Geometry: final body of the model. Coordinates: model frame, mm. A direction names the side the tool comes from. Give positions to 0.01 mm unless a question says otherwise; leave off trailing zeros. Order: outer loops, then holes, each group sorted by start corner. A loop starts at its lowest first (then second) coordinate and runs counter-clockwise, first axis right, second up. Notation, with made-up numbers: M 6.25,57 L 39.25,57 A12 cw 39.25,71 Z; hole C 42,88 d9. An arc over 180 degrees is marked long. Write item = value, one per line. Start each with the question number.
from build123d import *

# Parameters (mm, degrees)
SKETCH_1_W                         = 182.5
SKETCH_1_H                         = 55
SM_BASE_FLANGE_1_DEPTH             = 2
SM_EDGE_FLANGE_1_STRIP_W           = 9.4732
SM_EDGE_FLANGE_1_STRIP_H           = 2
SM_EDGE_FLANGE_1_STRIP_CUT_DEPTH   = 55
SM_EDGE_FLANGE_1_STRIP_2_W         = 9.4732
SM_EDGE_FLANGE_1_STRIP_2_H         = 2
SM_EDGE_FLANGE_1_STRIP_CUT_2_DEPTH = 55
SM_EDGE_FLANGE_1_DEPTH             = 55
SM_EDGE_FLANGE_1_BEND_DEPTH        = 55
SKETCH_12_W                        = 8
SKETCH_12_H                        = 7.5
CUT_EXTRUDE_1_DEPTH                = 10
FILLET_1_R                         = 2
SKETCH_13_R                        = 1.6
CUT_EXTRUDE_2_DEPTH                = 197
SKETCH_14_R                        = 1.6
CUT_EXTRUDE_3_DEPTH                = 10


# Sheet-metal steps are written as plain solids
with BuildPart() as part:
    # Sketch 1 → Базовая кромка1 (new body)
    with BuildSketch(Plane.XY):
        Rectangle(SKETCH_1_W, SKETCH_1_H)
    extrude(amount=-SM_BASE_FLANGE_1_DEPTH)

    # Ребро-кромка1 strip (across the edge) → Ребро-кромка1 strip cut (cut)
    with BuildSketch(Plane(origin=(-91.25, 27.5, 0), x_dir=(1, 0, 0), z_dir=(0, -1, 0))):
        with Locations((-2, -1)):
            Rectangle(SM_EDGE_FLANGE_1_STRIP_W, SM_EDGE_FLANGE_1_STRIP_H)
    extrude(amount=SM_EDGE_FLANGE_1_STRIP_CUT_DEPTH, mode=Mode.SUBTRACT)

    # Ребро-кромка1 strip 2 (across the edge) → Ребро-кромка1 strip cut 2 (cut)
    with BuildSketch(Plane(origin=(91.25, -27.5, 0), x_dir=(-1, 0, 0), z_dir=(0, 1, 0))):
        with Locations((-2, -1)):
            Rectangle(SM_EDGE_FLANGE_1_STRIP_2_W, SM_EDGE_FLANGE_1_STRIP_2_H)
    extrude(amount=SM_EDGE_FLANGE_1_STRIP_CUT_2_DEPTH, mode=Mode.SUBTRACT)

    # Ребро-кромка1 section (across the edge) → Ребро-кромка1 (add)
    with BuildSketch(Plane(origin=(-91.25, 27.5, 0), x_dir=(1, 0, 0), z_dir=(0, -1, 0))):
        with BuildLine():
            Line((0, 0.7366), (0, 28))
            Line((0, 28), (2, 28))
            Line((2, 28), (2, 0.7366))
            ThreePointArc((2, 0.7366), (2.215745145, 0.215745145), (2.7366, 0))
            Line((2.7366, 0), (2.7366, -2))
            ThreePointArc((2.7366, -2), (0.801531583, -1.198468417), (0, 0.7366))
        make_face()
    extrude(amount=SM_EDGE_FLANGE_1_DEPTH)

    # Ребро-кромка1 section 2 (across the edge) → Ребро-кромка1 bend (add)
    with BuildSketch(Plane(origin=(91.25, -27.5, 0), x_dir=(-1, 0, 0), z_dir=(0, 1, 0))):
        with BuildLine():
            Line((0, 0.7366), (0, 28))
            Line((0, 28), (2, 28))
            Line((2, 28), (2, 0.7366))
            ThreePointArc((2, 0.7366), (2.215745145, 0.215745145), (2.7366, 0))
            Line((2.7366, 0), (2.7366, -2))
            ThreePointArc((2.7366, -2), (0.801531583, -1.198468417), (0, 0.7366))
        make_face()
    extrude(amount=SM_EDGE_FLANGE_1_BEND_DEPTH)

    # Эскиз12 → Вырез-Вытянуть1 (cut)
    with BuildSketch(Plane.XY):
        with Locations((0, 23.75)):
            Rectangle(SKETCH_12_W, SKETCH_12_H)
        with Locations((30, 23.75)):
            Rectangle(SKETCH_12_W, SKETCH_12_H)
        with Locations((-30, 23.75)):
            Rectangle(SKETCH_12_W, SKETCH_12_H)
        with Locations((-60, 23.75)):
            Rectangle(SKETCH_12_W, SKETCH_12_H)
    extrude(amount=-CUT_EXTRUDE_1_DEPTH, mode=Mode.SUBTRACT)

    # Скругление1
    fillet_1_edges = [part.edges().sort_by_distance(p)[0] for p in [
        (-56, 20, -1),
        (-64, 20, -1),
        (-26, 20, -1),
        (-34, 20, -1),
        (34, 20, -1),
        (26, 20, -1),
        (4, 20, -1),
        (-4, 20, -1),
    ]]
    fillet(fillet_1_edges, radius=FILLET_1_R)

    # Эскиз13 → Вырез-Вытянуть2 (cut)
    with BuildSketch(Plane(origin=(91.25, 0, 0), x_dir=(0, 0, -1), z_dir=(1, 0, 0))):
        with Locations((-20.5, -20)):
            Circle(SKETCH_13_R)
        with Locations((-20.5, 22)):
            Circle(SKETCH_13_R)
    extrude(amount=-CUT_EXTRUDE_2_DEPTH, mode=Mode.SUBTRACT)

    # Эскиз14 → Вырез-Вытянуть3 (cut)
    with BuildSketch(Plane(origin=(0, 0, -2), x_dir=(-1, 0, 0), z_dir=(0, 0, -1))):
        with Locations((-63.25, 15.5)):
            Circle(SKETCH_14_R)
        with Locations((-63.25, -9.5)):
            Circle(SKETCH_14_R)
    extrude(amount=-CUT_EXTRUDE_3_DEPTH, mode=Mode.SUBTRACT)


solid = part.part
1) Cut plane C-C (y = -9.5). Return loops of the section in (x, z).
2) Ray query, L1, parallel to Y at x = -90.75, z = 20.5; L2, parallel to X at y = 7.5, z = 23.25; L3, parallel to Z at x = -8, y = 8. Return the intervals inside material, ascending.
3) Cut plane B-B (y = -20). Return loops of the section in (x, z).
4) Draft query along X for faces 3 (the flat face through (-91.25, 0, 14)), 4 (the cylindrical face through (90.264, -18.414, 20.708)), 5 (the flat face through (-1, 0, 0)). Return one class per face: pulls with the +X half, pulls with the -X half, needs draft (parallel to the pull), parting line crosses it, or undercut.
5) Pin query (flat end, axial travel): pin 1 Ø1.9 at (x, y) = (63.25, -9.5) entering from -Z; pin 2 Ø1 at (y, z) = (24, -1.5) entering from -X; pin 3 Ø2 at (y, z) = (23.5, -1) entering from +X; pin 4 Ø1.6 at (x, z) = (-61, -1) entering from +Y. Return the tip coordinate at first contact, or that it passes through.
6) Access query for faces 1 (the cylindrical face through (90.264, 23.586, 20.708)), 2 (the flat face through (-89.25, 0, 15)). Directions: +Z, -Z, +X, -X, +Y, -Y. A direction counts if a zero-diameter tool reaches every point of the face in a straight line with its end or side. Return the directions, or none.
7) Cut plane D-D (x = 63.25). Return loops of the section in (y, z).
8) Cut plane A-A (z = 15.25). Return loops of the section in (x, y).
Reply:
q1.outline = M -91.25,0.74 A2.74 ccw -88.51,-2 L 61.65,-2 L 61.65,0 L -88.51,0 A0.74 cw -89.25,0.74 L -89.25,28 L -91.25,28 Z; M 64.85,-2 L 88.51,-2 A2.74 ccw 91.25,0.74 L 91.25,28 L 89.25,28 L 89.25,0.74 A0.74 cw 88.51,0 L 64.85,0 Z
q2.L1 = -27.5 to -21.6, -18.4 to 20.4, 23.6 to 27.5
q2.L2 = -91.25 to -89.25, 89.25 to 91.25
q2.L3 = -2 to 0
q3.outline = M -91.25,0.74 A2.74 ccw -88.51,-2 L 88.51,-2 A2.74 ccw 91.25,0.74 L 91.25,18.9 L 89.25,18.9 L 89.25,0.74 A0.74 cw 88.51,0 L -88.51,0 A0.74 cw -89.25,0.74 L -89.25,18.9 L -91.25,18.9 Z; M -91.25,22.1 L -89.25,22.1 L -89.25,28 L -91.25,28 Z; M 89.25,22.1 L 91.25,22.1 L 91.25,28 L 89.25,28 Z
q4.face_3 = pulls with the -X half
q4.face_4 = needs draft
q4.face_5 = undercut
q5.pin_1 = through
q5.pin_2 = -90.63
q5.pin_3 = 91.15
q5.pin_4 = 20
q6.face_1 = +X, -X
q6.face_2 = +Z, +Y, -Y
q7.outline = M -27.5,-2 L -11.1,-2 L -11.1,0 L -27.5,0 Z; M -7.9,-2 L 13.9,-2 L 13.9,0 L -7.9,0 Z; M 17.1,-2 L 27.5,-2 L 27.5,0 L 17.1,0 Z
q8.outline = M -91.25,-27.5 L -89.25,-27.5 L -89.25,27.5 L -91.25,27.5 Z; M 89.25,-27.5 L 91.25,-27.5 L 91.25,27.5 L 89.25,27.5 Z
